For this review, take the finished solid that the model builds, in its own axes (mm). Face numbers are marked on the shaded views. Give positions to 0.01 mm unless a question says otherwise; leave off trailing zeros. Loops run counter-clockwise (first coordinate to the right, second up) from the corner with the lowest first, then second, coordinate; pieces in that order, holes last. Notation, with made-up numbers: (35, 79.5) - (40, 79.5) arc R19 ccw to (40, 95.5) - close; hole circle Ø7 at (89.25, 42). An arc over 180 degrees is marked (long way). Answer as CSV lines item,"result".
Autodesk Inventor part; units mm, degrees
ref_plane "YZ Plane" through (0, 0, 0) normal (1, 0, 0) x (0, 1, 0)
ref_plane "XZ Plane" through (0, 0, 0) normal (0, 1, 0) x (-1, 0, 0)
ref_plane "XY Plane" through (0, 0, 0) normal (0, 0, 1) x (1, 0, 0)
sketch "Sketch1" plane through (0, 0, 0) normal (0, 1, 0) x (-1, 0, 0)
  line L0 (0, 0) -> (34.925, 0)
  line L1 (38.1, -3.175) -> (38.1, -22.225)
  line L2 (34.925, -25.4) -> (0, -25.4)
  line L3 (0, -25.4) -> (0, 0)
  line L4 (0, 0) -> (0, -12.7)
  line L5 (0, -12.7) -> (25.4, -12.7)
  arc A0 (34.925, -25.4) -> (38.1, -22.225) centre (34.925, -22.225) ccw
  arc A1 (38.1, -3.175) -> (34.925, 0) centre (34.925, -3.175) ccw
  point P0 (38.1, -25.4)
  point P1 (38.1, 0)
  dimension "d0" = 38.1
  dimension "d1" = 25.4
  dimension "d2" = 12.7
  dimension "d3" = 25.4
  dimension "d7" = 3.175
extrude "Extrusion1" add sketch "Sketch1" along normal blind 3.175
hole "Hole1" at (-25.4, 0, -12.7) direction (0, 1, 0) diameter 5.1054 end through all
properties part number "1" material "Steel"
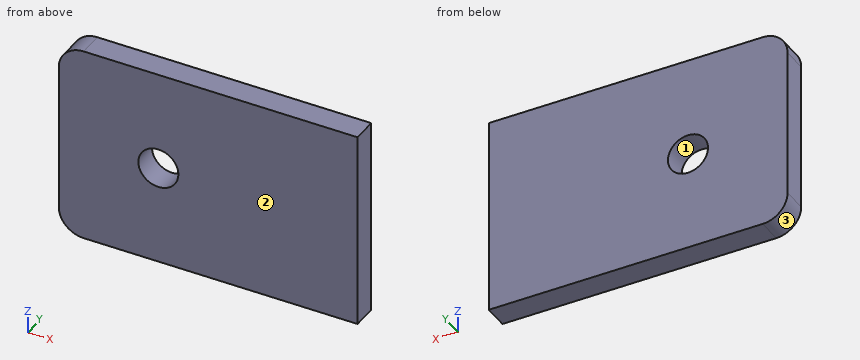
1) Consider section A-A on y = 0.95. Write out the cut boundary in (x, z) (3 decimals).
From the geometry:
outline,"(-38.1, -22.225) arc R3.175 ccw to (-34.925, -25.4) - (0, -25.4) - (0, 0) - (-34.925, 0) arc R3.175 ccw to (-38.1, -3.175) - close; hole circle Ø5.105 at (-25.4, -12.7)"
2) Consider section C-C on z = -12.7. Write out the cut boundary in (x, y) (3 decimals), and give its area (3 significant figures).
From the geometry:
outline,"(-38.1, 0) - (-27.953, 0) - (-27.953, 3.175) - (-38.1, 3.175) - close; (-22.847, 0) - (0, 0) - (0, 3.175) - (-22.847, 3.175) - close"
area,"105 mm^2"
3) Consider section B-B on x = -25.4. Write out the cut boundary in (y, z) (3 decimals).
From the geometry:
outline,"(0, -25.4) - (3.175, -25.4) - (3.175, -15.253) - (0, -15.253) - close; (0, -10.147) - (3.175, -10.147) - (3.175, 0) - (0, 0) - close"
4) Draft analysis for pull direction X (two halves, no side actions). For the marked faces 1, 2 and 3, state which applies: pulls with the +X half, pulls with the -X half, needs draft (parallel to the pull), parting line crosses it, or undercut.
From the geometry:
face 1,"undercut"
face 2,"needs draft"
face 3,"pulls with the -X half"
5) Wall thickness on line 1 (Z direction, x = -25.4, y = 1.05); line 2 (X direction, y = 1.8, z = -12.7); line 3 (X direction, y = 0.3, z = -12.5): over which ranges is each line inside the solid? List them lowest first. Write a range as from..to.
From the geometry:
line 1,"z = -25.4..-15.25, -10.15..0"
line 2,"x = -38.1..-27.95, -22.85..0"
line 3,"x = -38.1..-27.94, -22.86..0"
